Study the drawing (mm; zero at the part's minimum x, y, z) and answer. A direction names the side the tool comes from. Coordinates: 2 decimals unless noted, no trailing zeros. Write each loop counter-clockwise with the first axis right and the second up, starting at its lowest first coordinate (ties: lowest second). Pieces come first, ordered by that corner, then holes. Notation, with made-up numbers: M 32.25,86 L 74.25,86 A29 ccw 74.25,112 Z; hole C -1,-17.5 d9. An arc over 180 degrees is marked long. Answer as a JSON object with one key per item and string values. Group by question number.
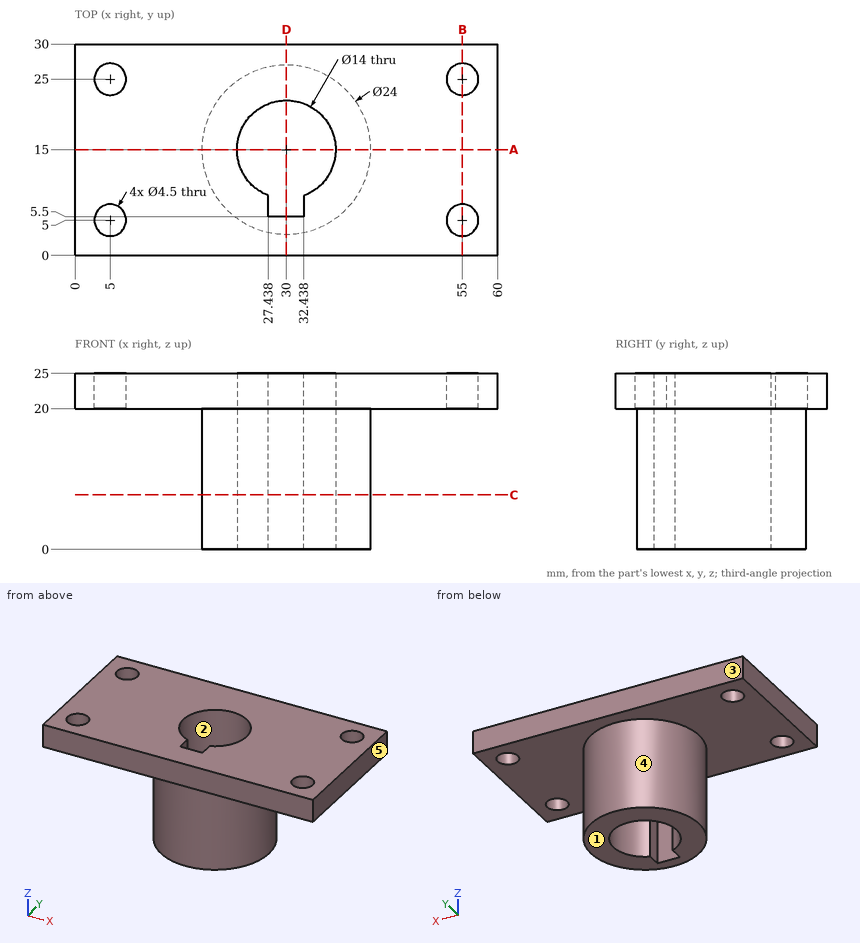
Item 1: A cutting plane is placed at A-A, the plane y = 15. Write down the section's boundary in (x, z), and give its area (3 significant figures).
Item 2: A cutting plane is placed at D-D, the plane x = 30. Write down the section's boundary in (y, z).
Item 3: A cutting plane is placed at C-C, the plane z = 7.75. Write down the section's boundary in (x, y), and give its area (3 significant figures).
Item 4: Flat-ended cylindrical pins translate along their axes: pin 1 Ø1 at (x, z) = (38.5, 10) entering from -Y; pin 2 Ø1.5 at (y, z) = (7.5, 10.5) entering from +X; pin 3 Ø5 at (x, y) = (5, 5) entering from -Z. Find the tip coordinate at first contact, or state that the pin passes through.
Item 5: A cutting plane is placed at B-B, the plane x = 55. Write down the section's boundary in (y, z), and give its area (3 significant figures).
Item 6: A tool of negligible diameter and unlimited length cuts with its end or side. For the marked faces 4 and 5, from which of +Z, -Z, +X, -X, +Y, -Y can it reach the whole face along a straight path? Write none if from no direction.
Item 7: Consider L1, parallel to Y at x = 5, z = 23.4; L2, parallel to X at y = 5, z = 22.15; L3, parallel to Y at x = 30, z = 14.25. Determine where each line is inside the solid, lowest interval first. Write a range as from..to.
Item 8: For a pull along Y with two mould halves and no side action, classify the marked faces 1, 2 and 3 as +Y half, -Y half, draft (parallel to the pull), parting line (faces both ways), or undercut.
Answer:
{
 "1": {"outline": "M 0,20 L 18,20 L 18,0 L 23,0 L 23,25 L 0,25 Z; M 37,0 L 42,0 L 42,20 L 60,20 L 60,25 L 37,25 Z", "area": "430 mm2"},
 "2": {"outline": "M 0,20 L 3,20 L 3,0 L 5.5,0 L 5.5,25 L 0,25 Z; M 22,0 L 27,0 L 27,20 L 30,20 L 30,25 L 22,25 Z"},
 "3": {"outline": "C 30,15 d24; hole M 27.44,5.5 L 32.44,5.5 L 32.44,8.44 A7 ccw long 27.44,8.49 Z", "area": "285 mm2"},
 "4": {"pin 1": "y = 6.06", "pin 2": "x = 39.92", "pin 3": "z = 20"},
 "5": {"outline": "M 0,20 L 2.75,20 L 2.75,25 L 0,25 Z; M 7.25,20 L 22.75,20 L 22.75,25 L 7.25,25 Z; M 27.25,20 L 30,20 L 30,25 L 27.25,25 Z", "area": "105 mm2"},
 "6": {"face 4": "-Z", "face 5": "+Z, -Z, +X, +Y, -Y"},
 "7": {"L1": "0..2.75, 7.25..22.75, 27.25..30", "L2": "0..2.75, 7.25..52.75, 57.25..60", "L3": "3..5.5, 22..27"},
 "8": {"face 1": "draft", "face 2": "undercut", "face 3": "+Y half"}
}
